Check sheet for the modelled part. Datum: model origin and axes. Units: mm. A direction names the side the tool comes from. Give positions to 0.01 mm unless a question says otherwise; leave off trailing zeros. Order: outer loops, then holes, each group sorted by start corner. A loop starts at its lowest first (then second) coordinate and runs counter-clockwise, first axis right, second up.
```python
from build123d import *

# Parameters (mm, degrees)
PAD004_DEPTH    = 32
POCKET005_DEPTH = 32
POCKET006_DEPTH = 16


with BuildPart() as part:
    # Sketch009 → Pad004 (new body)
    with BuildSketch(Plane.XY):
        with BuildLine():
            Line((-324, 84), (324, 84))
            ThreePointArc((360, 48), (349.455844, 73.455844), (324, 84))
            Line((360, 48), (360, 0))
            Line((360, 0), (-360, 0))
            Line((-360, 0), (-360, 48))
            ThreePointArc((-324, 84), (-349.455844, 73.455844), (-360, 48))
        make_face()
    extrude(amount=PAD004_DEPTH)

    # Sketch010 → Pocket005 (cut)
    with BuildSketch(Plane.XY.offset(32)):
        with BuildLine():
            ThreePointArc((-104.2, 46.2), (-108.4, 42), (-104.2, 37.8))
            Line((-104.2, 37.8), (-95.8, 37.8))
            ThreePointArc((-95.8, 37.8), (-91.6, 42), (-95.8, 46.2))
            Line((-95.8, 46.2), (-104.2, 46.2))
        make_face()
    pocket005 = extrude(amount=-POCKET005_DEPTH, mode=Mode.SUBTRACT)

    # Mirrored: Pocket005 across Sketch010 V_Axis
    add(pocket005.mirror(Plane(origin=(0, 0, 32), x_dir=(0, 0, 1), z_dir=(1, 0, 0))), mode=Mode.SUBTRACT)

    # Sketch011 → Pocket006 (cut)
    with BuildSketch(Plane(origin=(0, 0, 0), x_dir=(1, 0, 0), z_dir=(0, 0, -1))):
        with BuildLine():
            Line((-22.5, 0), (22.5, 0))
            Line((22.5, 0), (22.5, -57))
            ThreePointArc((16.5, -63), (20.742641, -61.242641), (22.5, -57))
            Line((16.5, -63), (-16.5, -63))
            ThreePointArc((-22.5, -57), (-20.742641, -61.242641), (-16.5, -63))
            Line((-22.5, -57), (-22.5, 0))
        make_face()
    extrude(amount=-POCKET006_DEPTH, mode=Mode.SUBTRACT)


solid = part.part
```
(1) Set-up check for faces 1 (the face through (22.5, 28, 8)), 2 (the face through (-360, 24, 16)): record each of +Z, -Z, +X, -X, +Y, -Y from which the full face is reachable in a straight line by a thin tool's end or side.
Response values:
face 1: -Z, -Y
face 2: +Z, -Z, -X, +Y, -Y
(2) Cross-section at B-B on y = 13. Enter the section's corners in (x, z), then the cut area to 3 significant figures.
Response values:
outline: (-360, 0) - (-22.5, 0) - (-22.5, 16) - (22.5, 16) - (22.5, 0) - (360, 0) - (360, 32) - (-360, 32) - close
area: 22,300 mm2
(3) Gauge pin test, flat ends, axial feed: pin 1 Ø17.5 at (x, z) = (3, 10) entering from -Y; pin 2 Ø10 at (y, z) = (68, 4) entering from -X; pin 3 Ø22.5 at (x, y) = (-7, 32.5) entering from -Z. Record the tip position at first contact, or that the pin passes through.
Response values:
pin 1: stops at y = 0
pin 2: stops at x = -356.73
pin 3: stops at z = 16
(4) Release check for a two-part mould opening along X. For faces 3 (the face through (-22.5, 29, 8)), 4 (the face through (5, 0, 19)), 5 (the face through (-349.174, 73.734, 15.776)) record: released by +X, released by -X, zero draft, split by the parting line, or undercut.
Response values:
face 3: undercut
face 4: zero draft
face 5: released by -X
(5) Cross-section at A-A on z = 6.5. Enter the section's corners in (x, y), then the cut area to 3 significant figures.
Response values:
outline: (-360, 0) - (-22.5, 0) - (-22.5, 57) arc R6 cw to (-16.5, 63) - (16.5, 63) arc R6 cw to (22.5, 57) - (22.5, 0) - (360, 0) - (360, 48) arc R36 ccw to (324, 84) - (-324, 84) arc R36 ccw to (-360, 48) - close; hole (-104.2, 37.8) - (-95.8, 37.8) arc R4.2 ccw to (-95.8, 46.2) - (-104.2, 46.2) arc R4.2 ccw to start; hole (95.8, 37.8) - (104.2, 37.8) arc R4.2 ccw to (104.2, 46.2) - (95.8, 46.2) arc R4.2 ccw to start
area: 56,900 mm2
(6) Material ranges on L1, parallel to X at y = 42, z = 24; L2, parallel to X at y = 36, z = 7; L3, parallel to X at y = 55, z = 4.5, recorded low to high.
Response values:
L1: x = -360 to -108.4, -91.6 to 91.6, 108.4 to 360
L2: x = -360 to -22.5, 22.5 to 360
L3: x = -359.31 to -22.5, 22.5 to 359.31
